Autodesk Inventor part; units mm, degrees
ref_plane "YZ Plane" through (0, 0, 0) normal (1, 0, 0) x (0, 1, 0)
ref_plane "XZ Plane" through (0, 0, 0) normal (0, 1, 0) x (-1, 0, 0)
ref_plane "XY Plane" through (0, 0, 0) normal (0, 0, 1) x (1, 0, 0)
sketch "Sketch1" plane through (0, 0, 0) normal (1, 0, 0) x (0, 1, 0)
  line L0 (0, 0) -> (50.8, 0)
  line L1 (50.8, 0) -> (50.8, -3.175)
  line L2 (50.8, -3.175) -> (0, -3.175)
  line L3 (0, -3.175) -> (0, 0)
  line L4 (0, 0) -> (3.175, 0)
  line L5 (3.175, 0) -> (3.175, -50.8)
  line L6 (3.175, -50.8) -> (0, -50.8)
  line L7 (0, -50.8) -> (0, 0)
  dimension "d0" = 50.8
  dimension "d1" = 3.175
  dimension "d2" = 3.175
  dimension "d3" = 50.8
extrude "Extrusion1" add sketch "Sketch1" along normal blind 25.4
fillet "Fillet1" radius 6.35 1 edges at (12.7, 3.175, -3.175)
hole "Hole1" at (12.7, 0, -12.7) direction (0, 1, 0) diameter 6.35 end through all
hole "Hole2" at (12.7, 0, -38.1) direction (0, 1, 0) diameter 6.35 end through all
hole "Hole3" at (12.7, 12.7, 0) direction (0, 0, -1) diameter 6.35 end through all
hole "Hole4" at (12.7, 38.1, 0) direction (0, 0, -1) diameter 6.35 end through all
properties part number "2in 4-hole Bracket 0.25in Hole"
Here's how the part is built. I have some questions about the finished solid (model axes, mm). A direction names the side the tool comes from. Round coordinates to 2 decimals unless told otherwise and drop trailing zeros. Order: outer loops, then holes, each group sorted by start corner. A loop starts at its lowest first (then second) coordinate and runs counter-clockwise, first axis right, second up. Notation, with made-up numbers: (-6, -18.5) -> (1, -18.5) arc R16 cw to (1, -4.5) -> close; hole circle Ø1 at (87.25, -38). An arc over 180 degrees is marked (long way). Use a Markdown table: item, result. Add a question column.
(1) For faces 1 (the face through (13, 0, -26)), 2 (the face through (13, 30, -3.175)), which set-ups out of +Z, -Z, +X, -X, +Y, -Y let a thin tool reach every point of the face, with its end or its side?
(2) I need wall thicknesses on line 1 along Z through (x, y) = (12.7, 2.3) (3 decimals); line 2 along X through (y, z) = (38, -1); line 3 along Y through (x, z) = (20.75, -43) (3 decimals). Which ranges of each line are inside material? Lowest first, please.
(3) Suppose I cut it at A-A, the plane z = -12.7. Please give me the cut outline in (x, y) (3 decimals), and give its area (3 significant figures).
(4) If we mould it in two halves opening along Y, with no side actions, what happens to faces 3 (the face through (13, 50.8, -2)), 4 (the face through (15.5, 11.2, -1.6)), 5 (the face through (14.63, 1.61, -10.18))? For each: released by +Y, released by -Y, zero draft, split by the parting line, or undercut.
(5) For pin 1 Ø1.5 at (x, z) = (11.5, -28.5) entering from +Y (3 decimals); pin 2 Ø6 at (x, z) = (23, -9) entering from -Y; pin 3 Ø8.5 at (x, y) = (12.7, 12.7) entering from -Z; pin 4 Ø4 at (x, y) = (22.5, 45.5) entering from -Z (3 decimals), each with a flat end and sliding along its axis, tell me the tip position at first contact or that it passes through.
(6) Suppose I cut it at C-C, the plane x = 8.5. Please give me the cut outline in (y, z) (3 decimals).
(7) Suppose I cut it at D-D, the plane x = 11.75. Please give me the cut outline in (y, z) (3 decimals), and give its area (3 significant figures).
(8) Suppose I cut it at B-B, the plane y = 12.7. Please give me the cut outline in (x, z) (3 decimals).
Verdict:
| question | item | result |
|---|---|---|
| 1 | face 1 | +Z, -Z, +X, -X, -Y |
| 1 | face 2 | -Z, +X, -X, +Y |
| 2 | line 1 | -50.8 to -41.275, -34.925 to -15.875, -9.525 to 0 |
| 2 | line 2 | 0 to 9.53, 15.87 to 25.4 |
| 2 | line 3 | 0 to 3.175 |
| 3 | outline | (0, 0) -> (9.525, 0) -> (9.525, 3.175) -> (0, 3.175) -> close; (15.875, 0) -> (25.4, 0) -> (25.4, 3.175) -> (15.875, 3.175) -> close |
| 3 | area | 60.5 mm2 |
| 4 | face 3 | released by +Y |
| 4 | face 4 | undercut |
| 4 | face 5 | zero draft |
| 5 | pin 1 | y = 3.175 |
| 5 | pin 2 | y = 0 |
| 5 | pin 3 | z = -3.27 |
| 5 | pin 4 | z = -3.175 |
| 6 | outline | (0, -50.8) -> (3.175, -50.8) -> (3.175, -9.525) arc R6.35 cw to (9.525, -3.175) -> (50.8, -3.175) -> (50.8, 0) -> (0, 0) -> close |
| 7 | outline | (0, -50.8) -> (3.175, -50.8) -> (3.175, -41.13) -> (0, -41.13) -> close; (0, -35.07) -> (3.175, -35.07) -> (3.175, -15.73) -> (0, -15.73) -> close; (0, -9.67) -> (3.175, -9.67) -> (3.175, -9.525) arc R6.35 cw to (9.525, -3.175) -> (9.67, -3.175) -> (9.67, 0) -> (0, 0) -> close; (15.73, -3.175) -> (35.07, -3.175) -> (35.07, 0) -> (15.73, 0) -> close; (41.13, -3.175) -> (50.8, -3.175) -> (50.8, 0) -> (41.13, 0) -> close |
| 7 | area | 244 mm2 |
| 8 | outline | (0, -3.175) -> (9.525, -3.175) -> (9.525, 0) -> (0, 0) -> close; (15.875, -3.175) -> (25.4, -3.175) -> (25.4, 0) -> (15.875, 0) -> close |
